The listing builds one solid part. Answer for the finished solid, in the listing's coordinates (mm). A direction names the side the tool comes from. Give positions to 0.01 mm unless a question says otherwise; leave off trailing zeros. Order: outer loops, then holes, each group sorted by start corner. A loop starts at its lowest first (then second) coordinate and runs counter-clockwise, first axis right, second up. Notation, with made-up numbers: (-11.5, 23.5) - (-6.5, 23.5) arc R16 ccw to (-6.5, 41.5) - close; hole circle Ø9 at (59, -36.5). An arc over 180 degrees is marked (long way). Answer in a Markdown table with one row per item. Add a question column.
```python
from build123d import *

# Parameters (mm, degrees)
F1_DEPTH     = 127
F2_T         = -2.54
F3_DEPTH     = 25.4
F5_DEPTH     = 132.08
F6_T         = 2.54
F6_T3_DEPTH  = 219.8768545095
F6_T5_DEPTH  = 219.7282038274
F6_T7_DEPTH  = 7.62
F6_T9_DEPTH  = 11.7497509401
F6_T11_DEPTH = 127
F6_T13_DEPTH = 214.6456904056
F6_T15_DEPTH = 5.1599103922
F6_T17_DEPTH = 7.62
F6_T19_DEPTH = 15.4153889552
F6_T21_DEPTH = 214.7908212861
F6_T23_DEPTH = 5.2038284596
F6_T26_ANGLE = 90.000000001
F6_T28_ANGLE = 90.000000001
F6_T30_ANGLE = 90.000000001
F6_T32_ANGLE = 90.000000001
F6_T34_ANGLE = 90.000000001
F6_T36_ANGLE = 90.000000001
F6_T38_ANGLE = 90.000000001
F6_T40_ANGLE = 90.000000001
F8_DEPTH     = 20.32


# Not quite as in the source:
# - a shell that OpenCascade refuses in one call is made with other operations: the cavity is built on its own and cut out


with BuildPart() as f1:
    # F0 (on Top) → F1 (new body)
    with BuildSketch(Plane.XY):
        with BuildLine():
            Line((132.6601760626, 49.2479032969), (-31.0818792045, 49.2479032969))
            ThreePointArc((-31.0818792045, 49.2479032969), (-49.0423914466, 41.8084155391), (-56.4818792045, 23.8479032969))
            Line((-56.4818792045, 23.8479032969), (158.0601760626, 23.8479032969))
            ThreePointArc((158.0601760626, 23.8479032969), (150.6206883047, 41.8084155391), (132.6601760626, 49.2479032969))
        make_face()
        Polygon((158.0601760626, 23.8479032969), (-56.4818792045, 23.8479032969), (-56.4818792045, -2.4297900897), (158.0601760626, -3.4250394454), align=None)
        Polygon((158.0601760626, -3.4250394454), (-56.4818792045, -2.4297900897), (-56.4818792045, -28.7074834764), (158.0601760626, -28.7074834764), align=None)
        with BuildLine():
            Line((158.0601760626, -28.7074834764), (-56.4818792045, -28.7074834764))
            ThreePointArc((-56.4818792045, -28.7074834764), (-49.0423914466, -46.6679957185), (-31.0818792045, -54.1074834764))
            Line((-31.0818792045, -54.1074834764), (132.6601760626, -54.1074834764))
            ThreePointArc((132.6601760626, -54.1074834764), (150.6206883047, -46.6679957185), (158.0601760626, -28.7074834764))
        make_face()
    extrude(amount=F1_DEPTH)

    # F2: a shell. OpenCascade refuses it in one call, so the cavity is built on its own and cut out:
    # the body offset inwards by the wall thickness, plus a prism from it out through each open face.
    f2_core = offset(f1.part, amount=F2_T, mode=Mode.PRIVATE)
    f2_exits = [f2_core.faces().sort_by_distance(p)[0] for p in [
        (50.789148, -51.567483, 63.5),
    ]]
    add(f2_core, mode=Mode.SUBTRACT)
    extrude(f2_exits, amount=-F2_T, mode=Mode.SUBTRACT)

    # F3 (cut): a face of the model
    f3_faces = [f1.faces().sort_by_distance(p)[0] for p in [
        (50.789148429, 46.7079032969, 63.5),
    ]]
    extrude(f3_faces, amount=-F3_DEPTH, mode=Mode.SUBTRACT)

    # F4 (on face) → F5 (join)
    with BuildSketch(Plane(origin=(0, 0, 0), x_dir=(1, 0, 0), z_dir=(0, 0, -1))):
        Polygon((158.0601760626, 28.7074834764), (-56.4818792045, 21.957822144), (-56.4818792045, -23.8479032969), (158.0601760626, -13.3886858821), align=None)
    extrude(amount=-F5_DEPTH)

    # F6: shell of thickness 2.54, made by hand


with BuildPart() as f6_core1:
    # F6_t2: copy of F1
    add(f1.part)

    # the walls: a layer under each face that stays
    f6_faces = [f6_core1.faces().sort_by_distance(p)[0] for p in [
        (-49.0423914466, 41.8084155391, 63.5),
        (50.789148429, 31.3182945895, 127),
        (50.789148429, 18.6182945895, 129.54),
        (50.789148429, -2.4297900897, 132.08),
        (50.789148429, -25.3326528102, 129.54),
        (50.789148429, -38.0326528102, 127),
        (-49.0423914466, -46.6679957185, 63.5),
        (-31.0818792045, -52.8374834764, 63.5),
        (-47.2463402224, -44.8719444943, 63.5),
        (-53.9418792045, -25.3726080063, 63.5),
        (50.789148429, -25.3326528102, 63.5),
        (155.5201760626, -28.6675282803, 63.5),
        (148.8246370805, -44.8719444943, 63.5),
        (132.6601760626, -52.8374834764, 63.5),
        (50.789148429, -38.0726080063, 124.46),
        (50.789148429, -38.0726080063, 2.54),
        (50.789148429, -54.1074834764, 1.27),
        (50.789148429, -54.1074834764, 125.73),
        (150.6206883047, -46.6679957185, 63.5),
        (158.0601760626, -2.4297900897, 66.04),
        (150.6206883047, 41.8084155391, 63.5),
        (132.6601760626, 47.9779032969, 63.5),
        (50.789148429, 31.3802088193, 2.54),
        (-47.2463402224, 40.0123643149, 63.5),
        (-53.9418792045, 23.7859890671, 63.5),
        (50.789148429, 18.6182945895, 63.5),
        (155.5201760626, 18.6802088193, 63.5),
        (50.789148429, 31.3802088193, 124.46),
        (148.8246370805, 40.0123643149, 63.5),
        (-56.4818792045, -2.4297900897, 66.04),
        (50.789148429, 49.2479032969, 125.73),
        (-31.0818792045, 47.9779032969, 63.5),
        (50.789148429, 49.2479032969, 1.27),
    ]]
    thicken(f6_faces, amount=-F6_T, mode=Mode.SUBTRACT)

    # F6_s4 → F6_t3 (cut)
    with BuildSketch(Plane(origin=(159.571223823, -7.779314508, 0), x_dir=(0, 0, 1), z_dir=(-0.9988137664, 0.0486935316, 0))):
        Polygon((127.0254, 21.0947119453), (124.46, 21.0693119453), (124.46, 18.5293119453), (127, 18.5293119453), align=None)
    extrude(amount=F6_T3_DEPTH, mode=Mode.SUBTRACT)

    # F6_s6 → F6_t5 (cut)
    with BuildSketch(Plane(origin=(-58.2746464734, 1.8333660851, 0), x_dir=(0, 0, 1), z_dir=(0.9995054766, -0.0314452262, 0))):
        Polygon((127.0254, 23.7484489574), (127, 21.1830489574), (124.46, 21.1830489574), (124.46, 23.7230489574), align=None)
    extrude(amount=F6_T5_DEPTH, mode=Mode.SUBTRACT)

    # F6_s8 → F6_t7 (cut)
    with BuildSketch(Plane.XZ.offset(49.0274834764)):
        Polygon((-31.0564792045, 2.5654), (-33.6218792045, 2.54), (-33.6218792045, 0), (-31.0818792045, 0), align=None)
        Polygon((-31.0564792045, 124.4346), (-33.6218792045, 124.46), (-33.6218792045, 127), (-31.0818792045, 127), align=None)
        Polygon((132.6347760626, 2.5654), (135.2001760626, 2.54), (135.2001760626, 0), (132.6601760626, 0), align=None)
        Polygon((132.6347760626, 124.4346), (135.2001760626, 124.46), (135.2001760626, 127), (132.6601760626, 127), align=None)
    extrude(amount=F6_T7_DEPTH, mode=Mode.SUBTRACT)

    # F6_s10 → F6_t9 (cut)
    with BuildSketch(Plane.XZ.offset(19.4977325363)):
        Polygon((-53.9164792045, 2.5654), (-56.4818792045, 2.54), (-56.4818792045, 0), (-53.9418792045, 0), align=None)
        Polygon((-53.9164792045, 124.4346), (-56.4818792045, 124.46), (-56.4818792045, 127), (-53.9418792045, 127), align=None)
    extrude(amount=F6_T9_DEPTH, mode=Mode.SUBTRACT)

    # F6_s12 → F6_t11 (cut)
    with BuildSketch(Plane.XY):
        Polygon((-53.9172779133, -22.0631199754), (-56.4818792045, -22.0377325363), (-56.4818792045, -19.4165654331), (-53.8620083299, -19.4989886257), align=None)
        Polygon((155.4939773538, -28.6529605233), (155.6000469372, -26.0888291736), (158.0601760626, -26.1662267655), (158.0601760626, -28.6275730842), align=None)
        Polygon((-53.9152423888, 23.749444707), (-56.4818792045, 23.7240748373), (-56.4818792045, 21.3048866852), (-54.0655607747, 21.1870878706), align=None)
        Polygon((155.4960128783, 13.5378842114), (155.3964944924, 10.975527375), (158.0601760626, 10.8456692704), (158.0601760626, 13.5125143417), align=None)
    extrude(amount=F6_T11_DEPTH, mode=Mode.SUBTRACT)

    # F6_s14 → F6_t13 (cut)
    with BuildSketch(Plane(origin=(-55.7346464734, 1.7534556929, 0), x_dir=(0, 0, 1), z_dir=(0.9995054766, -0.0314452262, 0))):
        Polygon((124.4346, 23.7484489574), (124.46, 21.1830489574), (127, 21.1830489574), (127, 23.7230489574), align=None)
        Polygon((2.5654, 23.7484489574), (2.54, 21.1830489574), (0, 21.1830489574), (0, 23.7230489574), align=None)
    extrude(amount=F6_T13_DEPTH, mode=Mode.SUBTRACT)

    # F6_s16 → F6_t15 (cut)
    with BuildSketch(Plane.XZ.offset(26.0875730842)):
        Polygon((155.4947760626, 124.4346), (158.0601760626, 124.46), (158.0601760626, 127), (155.5201760626, 127), align=None)
        Polygon((155.4947760626, 2.5654), (158.0601760626, 2.54), (158.0601760626, 0), (155.5201760626, 0), align=None)
    extrude(amount=F6_T15_DEPTH, mode=Mode.SUBTRACT)

    # F6_s18 → F6_t17 (cut)
    with BuildSketch(Plane.XZ.offset(-51.7879032969)):
        Polygon((132.6347760626, 124.4346), (135.2001760626, 124.46), (135.2001760626, 127), (132.6601760626, 127), align=None)
        Polygon((132.6347760626, 2.5654), (135.2001760626, 2.54), (135.2001760626, 0), (132.6601760626, 0), align=None)
        Polygon((-31.0564792045, 2.5654), (-31.0818792045, 0), (-33.6218792045, 0), (-33.6218792045, 2.54), align=None)
        Polygon((-31.0564792045, 124.4346), (-31.0818792045, 127), (-33.6218792045, 127), (-33.6218792045, 124.46), align=None)
    extrude(amount=F6_T17_DEPTH, mode=Mode.SUBTRACT)

    # F6_s20 → F6_t19 (cut)
    with BuildSketch(Plane.XZ.offset(-26.3879032969)):
        Polygon((155.4947760626, 2.5654), (155.5201760626, 0), (158.0601760626, 0), (158.0601760626, 2.54), align=None)
        Polygon((155.4947760626, 124.4346), (158.0601760626, 124.46), (158.0601760626, 127), (155.5201760626, 127), align=None)
    extrude(amount=F6_T19_DEPTH, mode=Mode.SUBTRACT)

    # F6_s22 → F6_t21 (cut)
    with BuildSketch(Plane(origin=(157.031223823, -7.6554860484, 0), x_dir=(0, 0, 1), z_dir=(-0.9988137664, 0.0486935316, 0))):
        Polygon((2.5654, 21.0947119453), (0, 21.0693119453), (0, 18.5293119453), (2.54, 18.5293119453), align=None)
        Polygon((124.4346, 21.0947119453), (124.46, 18.5293119453), (127, 18.5293119453), (127, 21.0693119453), align=None)
    extrude(amount=F6_T21_DEPTH, mode=Mode.SUBTRACT)

    # F6_s24 → F6_t23 (cut)
    with BuildSketch(Plane.XZ.offset(-26.3879032969)):
        Polygon((-53.9164792045, 2.5654), (-53.9418792045, 0), (-56.4818792045, 0), (-56.4818792045, 2.54), align=None)
        Polygon((-53.9164792045, 124.4346), (-56.4818792045, 124.46), (-56.4818792045, 127), (-53.9418792045, 127), align=None)
    extrude(amount=F6_T23_DEPTH, mode=Mode.SUBTRACT)

    # F6_s25 → F6_t26 (revolve, cut)
    with BuildSketch(Plane.YZ.offset(-31.0818792045)):
        Polygon((-51.5420834764, 124.4346), (-54.1074834764, 124.46), (-54.1074834764, 127), (-51.5674834764, 127), align=None)
    revolve(axis=Axis((-31.0818792045, -28.7074834764, 124.46), (0, 0, -1)), revolution_arc=F6_T26_ANGLE, mode=Mode.SUBTRACT)

    # F6_s27 → F6_t28 (revolve, cut)
    with BuildSketch(Plane.YZ.offset(-31.0818792045)):
        Polygon((-51.5420834764, 2.5654), (-54.1074834764, 2.54), (-54.1074834764, 0), (-51.5674834764, 0), align=None)
    revolve(axis=Axis((-31.0818792045, -28.7074834764, 2.54), (0, 0, -1)), revolution_arc=F6_T28_ANGLE, mode=Mode.SUBTRACT)

    # F6_s29 → F6_t30 (revolve, cut)
    with BuildSketch(Plane.XZ.offset(28.7074834764)):
        Polygon((155.4947760626, 124.4346), (158.0601760626, 124.46), (158.0601760626, 127), (155.5201760626, 127), align=None)
    revolve(axis=Axis((132.6601760626, -28.7074834764, 124.46), (0, 0, -1)), revolution_arc=F6_T30_ANGLE, mode=Mode.SUBTRACT)

    # F6_s31 → F6_t32 (revolve, cut)
    with BuildSketch(Plane.XZ.offset(28.7074834764)):
        Polygon((155.4947760626, 2.5654), (158.0601760626, 2.54), (158.0601760626, 0), (155.5201760626, 0), align=None)
    revolve(axis=Axis((132.6601760626, -28.7074834764, 2.54), (0, 0, -1)), revolution_arc=F6_T32_ANGLE, mode=Mode.SUBTRACT)

    # F6_s33 → F6_t34 (revolve, cut)
    with BuildSketch(Plane.YZ.offset(132.6601760626)):
        Polygon((46.6825032969, 2.5654), (46.7079032969, 0), (49.2479032969, 0), (49.2479032969, 2.54), align=None)
    revolve(axis=Axis((132.6601760626, 23.8479032969, 2.54), (0, 0, -1)), revolution_arc=F6_T34_ANGLE, mode=Mode.SUBTRACT)

    # F6_s35 → F6_t36 (revolve, cut)
    with BuildSketch(Plane.XZ.offset(-23.8479032969)):
        Polygon((-53.9164792045, 2.5654), (-53.9418792045, 0), (-56.4818792045, 0), (-56.4818792045, 2.54), align=None)
    revolve(axis=Axis((-31.0818792045, 23.8479032969, 2.54), (0, 0, -1)), revolution_arc=F6_T36_ANGLE, mode=Mode.SUBTRACT)

    # F6_s37 → F6_t38 (revolve, cut)
    with BuildSketch(Plane.XZ.offset(-23.8479032969)):
        Polygon((-53.9164792045, 124.4346), (-56.4818792045, 124.46), (-56.4818792045, 127), (-53.9418792045, 127), align=None)
    revolve(axis=Axis((-31.0818792045, 23.8479032969, 124.46), (0, 0, -1)), revolution_arc=F6_T38_ANGLE, mode=Mode.SUBTRACT)

    # F6_s39 → F6_t40 (revolve, cut)
    with BuildSketch(Plane.YZ.offset(132.6601760626)):
        Polygon((46.6825032969, 124.4346), (46.7079032969, 127), (49.2479032969, 127), (49.2479032969, 124.46), align=None)
    revolve(axis=Axis((132.6601760626, 23.8479032969, 124.46), (0, 0, -1)), revolution_arc=F6_T40_ANGLE, mode=Mode.SUBTRACT)


with BuildPart() as f1_1:
    add(f1.part)

    # what is left inside the walls is the cavity
    f6_cavity = [f6_core1.part.solids().sort_by_distance(p)[0] for p in [
        (15.877569, 17.751835, 64.77),
    ]]
    add(f6_cavity, mode=Mode.SUBTRACT)

    # F7 (on face) → F8 (join)
    with BuildSketch(Plane.YZ.offset(158.0601760626)):
        Polygon((23.8479032969, -59.71023524), (23.8479032969, 0), (-28.7074834764, 0), (-28.7074834764, -29.3008414079), (-94.8645432204, -29.3008414079), (-94.8645432204, -59.71023524), align=None)
    extrude(amount=-F8_DEPTH)


solid = f1_1.part
```
(1) Find section A-A, the plane y = -42. Write down the section's boundary in (x, z).
(2) Each of these flat-tipped pins is pushed along its axis until it touches: P1, Ø23.5, axis at x = 38, y = -6, coming from the -Z side; P2, Ø8, axis at x = 30.5, y = -39.5, coming from the -Z side; P3, Ø3, axis at y = 47.5, z = 71, coming from the +X side. Where does it stop, or does it pass through?
(3) Straight lines are drawn through the part: line 1 (Z direction, x = 6.5, y = 31); line 2 (X direction, y = 2.5, z = 76.5); line 3 (Y direction, x = 72, z = 85). For each, find the intervals that lie inside material, in ascending order.
(4) The mould has two halves that part along X. Classify faces 1 (the face through (-49.24, -46.47, 62.61)), 2 (the face through (149.001, 39.834, 62.647)), 3 (the face through (150.422, -46.864, 62.611)): +X half, -X half, draft (parallel to the pull), parting line (faces both ways), or undercut.
(5) Find section B-B, the plane y = -9. Write down the section's boundary in (x, z).
(6) Find section D-D, the plane x = 90. Write down the section's boundary in (y, z) (3 decimals), plus the area to 3 significant figures.
(7) Find section C-C, the plane z = 20.5. Write down the section's boundary in (x, y), plus the area to 3 significant figures.
(8) For faces 4 (the face through (148, -28.707, -14)), 5 (the face through (49.29, 18.69, 129.5)), 6 (the face through (49, -38, 2.54)), 7 (the face through (137.74, -23, -36)), 8 (the face through (148, 23.848, -30)), determine the directions among +Z, -Z, +X, -X, +Y, -Y from which every point of the face is accessible in a straight line to the end or side of a thin tool.
Answer key:
| question | item | result |
|---|---|---|
| 1 | outline | (-52.73, 0) - (154.3, 0) - (154.3, 127) - (-52.73, 127) - close; (137.74, -59.71) - (158.06, -59.71) - (158.06, -29.3) - (137.74, -29.3) - close; hole (-49.68, 2.54) - (151.26, 2.54) - (151.26, 124.46) - (-49.68, 124.46) - close |
| 2 | P1 | z = 129.54 |
| 2 | P2 | z = 0 |
| 2 | P3 | x = 145.09 |
| 3 | line 1 | 0 to 2.54, 124.46 to 127 |
| 3 | line 2 | -56.48 to -53.94, 155.52 to 158.06 |
| 3 | line 3 | -26 to -23.46, 15.04 to 17.58 |
| 4 | face 1 | -X half |
| 4 | face 2 | undercut |
| 4 | face 3 | +X half |
| 5 | outline | (-56.48, 0) - (-53.94, 0) - (-53.94, 129.54) - (155.52, 129.54) - (155.52, 0) - (137.74, 0) - (137.74, -59.71) - (158.06, -59.71) - (158.06, 132.08) - (-56.48, 132.08) - close |
| 6 | outline | (-54.107, 0) - (-24.025, 0) - (-24.025, 129.54) - (14.164, 129.54) - (14.164, 0) - (49.248, 0) - (49.248, 2.54) - (16.707, 2.54) - (16.707, 124.46) - (49.248, 124.46) - (49.248, 127) - (16.707, 127) - (16.707, 132.08) - (-26.566, 132.08) - (-26.566, 127) - (-54.107, 127) - (-54.107, 124.46) - (-26.566, 124.46) - (-26.566, 2.54) - (-54.107, 2.54) - close |
| 6 | area | 1,070 mm² |
| 7 | outline | (-56.48, -28.71) arc R25.4 ccw to (-31.08, -54.11) - (-31.08, -51.57) arc R22.86 cw to (-53.94, -28.71) - (-53.94, -22.04) - (155.52, -28.63) - (155.52, -28.71) arc R22.86 cw to (132.66, -51.57) - (132.66, -54.11) arc R25.4 ccw to (158.06, -28.71) - (158.06, 23.85) arc R25.4 ccw to (132.66, 49.25) - (132.66, 46.71) arc R22.86 cw to (155.52, 23.85) - (155.52, 13.51) - (-53.94, 23.72) - (-53.94, 23.85) arc R22.86 cw to (-31.08, 46.71) - (-31.08, 49.25) arc R25.4 ccw to (-56.48, 23.85) - close; hole (-53.94, -19.5) - (155.52, -26.09) - (155.52, 10.97) - (-53.94, 21.18) - close |
| 7 | area | 1,720 mm² |
| 8 | face 4 | +X, -X, -Y |
| 8 | face 5 | +Z, +X, +Y |
| 8 | face 6 | none |
| 8 | face 7 | -Z, -X, +Y, -Y |
| 8 | face 8 | -Z, +X, -X, +Y |
